```python
from build123d import *

# Parameters (mm, degrees)
BOSS_EXTRUDE1_DEPTH = 30
SKETCH3_R           = 4
CUT_EXTRUDE1_DEPTH  = 30
CUT_EXTRUDE2_REACH  = 152.867
SKETCH5_W           = 24
SKETCH5_H           = 6


with BuildPart() as part:
    # Sketch1 → Revolve5 (revolve)
    with BuildSketch(Plane.XY, mode=Mode.PRIVATE) as revolve5_sk:
        with BuildLine():
            Line((0, 0), (60, 0))
            add(Edge.make_bspline(
                [(13.077250629, -110), (26.441462871, -105.381596251), (58.400000122, -57.571050955), (51.598678878, -21.794632863), (60, 0)],
                knots=[0.017667594, 0.017667594, 0.017667594, 0.017667594, 0.353401106, 1, 1, 1, 1], degree=3))
            ThreePointArc((13.077250629, -110), (8.624288133, -112.501880222), (5.3315658, -116.406526078))
            ThreePointArc((5.3315658, -116.406526078), (3.082984988, -118.82225748), (0, -120))
            Line((0, -120), (0, 0))
        make_face()
    revolve(revolve5_sk.sketch.rotate(Axis((0, 0, 0), (0, -1, 0)), 180), axis=Axis((0, 0, 0), (0, -1, 0)))

    # Sketch2 → Boss-Extrude1 (add)
    with BuildSketch(Plane(origin=(0, 0, 0), x_dir=(1, 0, 0), z_dir=(0, 1, 0))):
        with BuildLine():
            Line((12, 9), (12, -9))
            ThreePointArc((12, -9), (0, -15), (-12, -9))
            Line((-12, -9), (-12, 9))
            ThreePointArc((-12, 9), (0, 15), (12, 9))
        make_face()
    extrude(amount=BOSS_EXTRUDE1_DEPTH)

    # Sketch3 → Cut-Extrude1 (cut)
    with BuildSketch(Plane(origin=(0, 30, 0), x_dir=(1, 0, 0), z_dir=(0, 1, 0))):
        with Locations(Location((0, 0, 0), (0, 0, 270))):
            Circle(SKETCH3_R)
    extrude(amount=-CUT_EXTRUDE1_DEPTH, mode=Mode.SUBTRACT)

    # Sketch5 → Cut-Extrude2 (cut, up to next)
    with BuildSketch(Plane.XY.offset(9), mode=Mode.PRIVATE) as cut_extrude2_sk1:
        with Locations((0, 18)):
            Rectangle(SKETCH5_W, SKETCH5_H)
    cut_extrude2_tool1 = extrude(cut_extrude2_sk1.sketch, amount=CUT_EXTRUDE2_REACH, mode=Mode.PRIVATE) & part.part
    cut_extrude2 = cut_extrude2_tool1.solids().sort_by_distance((0, 18, 9))[0]
    add(cut_extrude2, mode=Mode.SUBTRACT)

    # Mirror1: Cut-Extrude2 across plane
    add(cut_extrude2.mirror(Plane.XY), mode=Mode.SUBTRACT)


solid = part.part
```
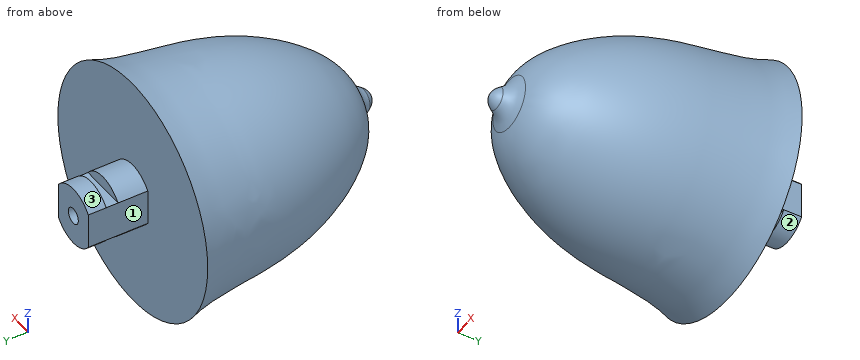
Read the model definition and answer for the solid it produces. Units are mm, in the model's axes. Face numbers are marked on the shaded views. A direction names the side the tool comes from. Give positions to 0.01 mm unless a question says otherwise; leave off trailing zeros. Answer in a Markdown table with one row per item.
1) Each of these flat-tipped pins is pushed along its axis until it touches: pin 1 Ø1.5 at (x, z) = (-17, -0.5) entering from -Y; pin 2 Ø6.5 at (x, z) = (0, 0) entering from +Y; pin 3 Ø5 at (y, z) = (-16.5, 37.5) entering from +X. Where does it stop, or does it pass through?
Results list:
| item | result |
|---|---|
| pin 1 | y = -108.66 |
| pin 2 | y = 0 |
| pin 3 | x = 43.39 |
2) Straight lines are drawn through the part: line 1 (X direction, y = 14.5, z = 0); line 2 (Y direction, x = 3, z = 10); line 3 (X direction, y = 4.5, z = -5). For each, find the intervals that lie inside material, in ascending order. Write a range as [from, to].
Results list:
| item | result |
|---|---|
| line 1 | [-12, -4], [4, 12] |
| line 2 | [-111.22, 15], [21, 30] |
| line 3 | [-12, 12] |
3) A tool of negligible diameter and unlimited length cuts with its end or side. For the marked faces 1, 2 and 3, from which of +Z, -Z, +X, -X, +Y, -Y can it reach the whole face along a straight path? Write none if from no direction.
Results list:
| item | result |
|---|---|
| face 1 | +Z, -Z, -X, +Y |
| face 2 | -Z, +Y |
| face 3 | +Z, +Y |
